Here's how the part is built. I have some questions about the finished solid (model axes, mm). Face numbers are marked on the shaded views. A direction names the side the tool comes from. Coordinates: 2 decimals unless noted, no trailing zeros. Order: outer loops, then holes, each group sorted by start corner. A loop starts at its lowest first (then second) coordinate and runs counter-clockwise, first axis right, second up. Notation, with made-up numbers: (-33.5, 60) - (-8.5, 60) arc R22 ccw to (-8.5, 95) - close; hole circle Ø1 at (-34, -14). An arc over 180 degrees is marked (long way). Answer in a Markdown table with one row per item. Add a question column.
Item 1: Thinking about a two-plate mould opening in Z: for the marked faces 1, 2, 3 and 4, which applies, +Z half, -Z half, draft (parallel to the pull), parting line (faces both ways), or undercut?
Item 2: Will these pins go through, and if not, where does the flat tip stop? pin 1 Ø1.8 at (y, z) = (6, 58) entering from -X; pin 2 Ø5 at (y, z) = (9.5, 51) entering from -X; pin 3 Ø10 at (y, z) = (-3.5, 6) entering from +X; pin 4 Ø5 at (y, z) = (-3, 50.5) entering from -X.
Item 3: On a 3-axis mill with a long thin cutter (end or side, diameter ignored), from which of +Z, -Z, +X, -X, +Y, -Y can I reach the whole of each face in a straight line? I mean the marked faces 5, 6 and 7. Say none if no direction works.
Item 4: I want a section at C-C (z = 21). Please give me the cut outline in (x, y).
Item 5: If I drill on line 1 along Z through (x, y) = (12.5, -16); line 2 along Y through (x, z) = (52, 57.5); line 3 along Z through (x, y) = (20.5, 2), over which ranges is the centre line in solid material (lowest first)? Write a range as from..to.
Item 6: I want a section at A-A (z = 30). Please give me the cut outline in (x, y), plus the area to 3 significant figures.
Item 7: I want a section at B-B (y = -5). Count the separate pieces of the cut face and the enclosed holes in it, plus the area to 3 significant figures.
```python
from build123d import *

# Parameters (mm, degrees)
BOSS_EXTRUDE1_DEPTH     = 60
CUT_EXTRUDE1_DEPTH      = 100
CUT_EXTRUDE1_DEPTH_BACK = 100
SKETCH2_R               = 7.5
CUT_EXTRUDE2_DEPTH      = 105.828431258
CUT_EXTRUDE3_DEPTH      = 105.828431258
CUT_EXTRUDE3_DEPTH_BACK = 105.828431258
SKETCH4_W               = 49
SKETCH4_H               = 32
CUT_EXTRUDE4_DEPTH      = 105.828431258
CUT_EXTRUDE4_DEPTH_BACK = 105.828431258
SKETCH5_W               = 16
SKETCH5_H               = 6
CUT_EXTRUDE6_DEPTH      = 100
CUT_EXTRUDE6_DEPTH_BACK = 100
SKETCH6_R               = 7
CUT_EXTRUDE7_DEPTH      = 6
CUT_EXTRUDE13_START     = -6
CUT_EXTRUDE13_OUTLINE_R = 7.5
CUT_EXTRUDE13_DEPTH     = 6


# Read off the part's stored shape, not the designer's step: Cut-Extrude13
with BuildPart() as part:
    # Sketch1 → Boss-Extrude1 (new body)
    with BuildSketch(Plane.XY):
        with BuildLine():
            Line((60, 18), (38.418745425, 18))
            ThreePointArc((38.418745425, 18), (17.205541989, 13.276925691), (0, 0))
            Line((0, 0), (0, -24))
            Line((0, -24), (60, -24))
            Line((60, -24), (75, -15.339745962))
            Line((75, -15.339745962), (75, 9.339745962))
            Line((75, 9.339745962), (60, 18))
        make_face()
    extrude(amount=BOSS_EXTRUDE1_DEPTH)

    # Sketch2 → Cut-Extrude1 (cut, two sides: drawn at the far end of the back side and taken through both)
    with BuildSketch(Plane.XY.offset(60).offset(-CUT_EXTRUDE1_DEPTH_BACK)):
        with Locations((29, -5)):
            Circle(SKETCH2_R)
    extrude(amount=CUT_EXTRUDE1_DEPTH + CUT_EXTRUDE1_DEPTH_BACK, mode=Mode.SUBTRACT)

    # Sketch3 → Cut-Extrude2 (cut, through all)
    with BuildSketch(Plane(origin=(0, 18, 0), x_dir=(1, 0, 0), z_dir=(0, 1, 0))):
        Polygon((60, 0), (75, -15), (75, 0), align=None)
        Polygon((60, -60), (75, -60), (75, -45), align=None)
    extrude(amount=-CUT_EXTRUDE2_DEPTH, mode=Mode.SUBTRACT)

    # Sketch4 → Cut-Extrude3 (cut, two sides: drawn at the far end of the back side and taken through both)
    with BuildSketch(Plane(origin=(0, 18, 0), x_dir=(1, 0, 0), z_dir=(0, 1, 0)).offset(-CUT_EXTRUDE3_DEPTH_BACK)):
        with Locations((24.5, -30)):
            Rectangle(SKETCH4_W, SKETCH4_H)
    extrude(amount=CUT_EXTRUDE3_DEPTH + CUT_EXTRUDE3_DEPTH_BACK, mode=Mode.SUBTRACT)

    # Sketch5 → Cut-Extrude4 (cut, two sides: drawn at the far end of the back side and taken through both)
    with BuildSketch(Plane(origin=(0, 18, 0), x_dir=(1, 0, 0), z_dir=(0, 1, 0)).offset(-CUT_EXTRUDE4_DEPTH_BACK)):
        with Locations((8, -11)):
            Rectangle(SKETCH5_W, SKETCH5_H)
        with Locations((8, -49)):
            Rectangle(SKETCH5_W, SKETCH5_H)
    extrude(amount=CUT_EXTRUDE4_DEPTH + CUT_EXTRUDE4_DEPTH_BACK, mode=Mode.SUBTRACT)

    # Sketch6 → Cut-Extrude6 (cut, two sides: drawn at the far end of the back side and taken through both)
    with BuildSketch(Plane(origin=(75, 0, 0), x_dir=(0, 0, -1), z_dir=(1, 0, 0)).offset(-CUT_EXTRUDE6_DEPTH_BACK)):
        with Locations((-30, -3)):
            Circle(SKETCH6_R)
    extrude(amount=CUT_EXTRUDE6_DEPTH + CUT_EXTRUDE6_DEPTH_BACK, mode=Mode.SUBTRACT)

    # 3DSketch1 → Cut-Extrude7 (cut)
    with BuildSketch(Plane(origin=(2, -22, 60), x_dir=(0.8274757743917585, 0.5615014183372646, 0), z_dir=(0, 0, -1))):
        with BuildLine():
            Line((0, 0), (46.338643366, 31.444079427))
            Line((46.338643366, 31.444079427), (67.675697263, 0))
            Line((67.675697263, 0), (51.472683469, -10.994902217))
            add(Edge.make_bspline(
                [(51.472683469, -10.994902217), (51.00988811, -11.308941925), (50.54709275, -11.622981633), (50.081937087, -11.933401281), (48.672308272, -12.842939856), (47.19895125, -13.654736784), (46.194725989, -14.158808627), (43.645035729, -15.341959521), (41.037130207, -16.372005027), (39.451628921, -16.928242653), (36.239509448, -17.903795074), (32.945954255, -18.578814885), (31.283999686, -18.84258235), (27.940100514, -19.225413824), (24.576949104, -19.324401234), (22.894937643, -19.299992929), (20.094000133, -19.130990082), (17.316239244, -18.739706134), (16.20712535, -18.550994584), (14.685796858, -18.252372423), (13.175745435, -17.907974305), (12.762523967, -17.809287194), (12.350651667, -17.705660499), (11.940378642, -17.596347472)],
                knots=[0, 0, 0, 0, 0, 0, 0.067720945, 0.067720945, 0.067720945, 0.203162835, 0.203162835, 0.203162835, 0.406325669, 0.406325669, 0.406325669, 0.609488504, 0.609488504, 0.609488504, 0.812651339, 0.812651339, 0.812651339, 0.94859619, 0.94859619, 0.94859619, 1, 1, 1, 1, 1, 1], degree=5))
            Line((11.940378642, -17.596347472), (8.989958239, -16.810238314))
            Line((8.989958239, -16.810238314), (-1.654951549, -1.123002837))
            Line((-1.654951549, -1.123002837), (0, 0))
        make_face()
    extrude(amount=CUT_EXTRUDE7_DEPTH, mode=Mode.SUBTRACT)

    # Cut-Extrude13 outline → Cut-Extrude13 (cut)
    with BuildSketch(Plane.XY.offset(54).offset(CUT_EXTRUDE13_START)):
        with BuildLine():
            Line((58, 16), (38.418745425, 16))
            add(Edge.make_bspline(
                [(38.418745425, 16), (37.859459734, 16), (37.300174044, 16), (36.740967929, 15.995679173), (35.063827034, 15.956791732), (33.388834665, 15.801241966), (32.274825535, 15.654475296), (29.500677707, 15.201849301), (26.764327053, 14.589844353), (25.140034933, 14.159856293), (23.537172375, 13.661674471), (21.959650667, 13.089890217)],
                knots=[0, 0, 0, 0, 0, 0, 0.067720945, 0.067720945, 0.067720945, 0.203162835, 0.203162835, 0.203162835, 0.406325669, 0.406325669, 0.406325669, 0.406325669, 0.406325669, 0.406325669], degree=5))
            ThreePointArc((21.959650667, 13.089890217), (19.961391414, 12.309435597), (18, 11.440474621))
            Line((18, 11.440474621), (18, -22))
            Line((18, -22), (58, -22))
            Line((58, -22), (58, 16))
        make_face()
        with Locations((29, -5)):
            Circle(CUT_EXTRUDE13_OUTLINE_R, mode=Mode.SUBTRACT)
    extrude(amount=CUT_EXTRUDE13_DEPTH, mode=Mode.SUBTRACT)


solid = part.part
```
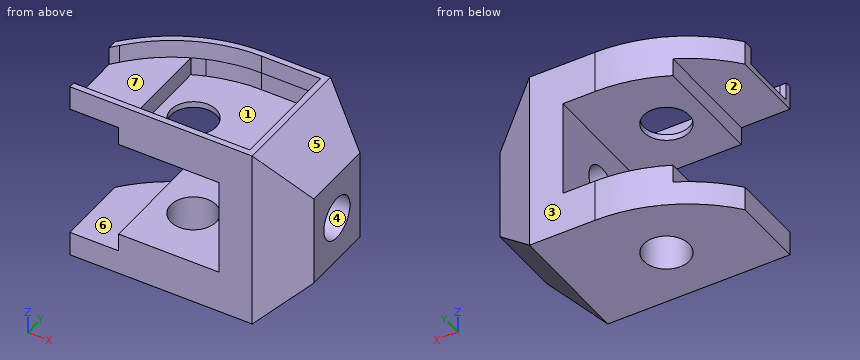
Values follow:
| question | item | result |
|---|---|---|
| 1 | face 1 | +Z half |
| 1 | face 2 | undercut |
| 1 | face 3 | draft |
| 1 | face 4 | undercut |
| 2 | pin 1 | stops at x = 4.9 |
| 2 | pin 2 | stops at x = 7.39 |
| 2 | pin 3 | stops at x = 71 |
| 2 | pin 4 | stops at x = 0 |
| 3 | face 5 | +Z, +X, +Y, -Y |
| 3 | face 6 | -X, +Y, -Y |
| 3 | face 7 | +Z |
| 4 | outline | (49, -24) - (60, -24) - (75, -15.34) - (75, 9.34) - (60, 18) - (49, 18) - close |
| 5 | line 1 | z = 0..8, 52..54 |
| 5 | line 2 | y = -24..-22, 16..18 |
| 5 | line 3 | z = 0..14, 46..48 |
| 6 | outline | (49, -24) - (60, -24) - (75, -15.34) - (75, -10) - (49, -10) - close; (49, 4) - (75, 4) - (75, 9.34) - (60, 18) - (49, 18) - close |
| 6 | area | 598 mm^2 |
| 7 | separate pieces | 4 |
| 7 | enclosed holes | 0 |
| 7 | area | 1,340 mm^2 |
